Check sheet for the modelled part. Datum: model origin and axes. Units: mm. A direction names the side the tool comes from. Coordinates: 2 decimals unless noted, no trailing zeros. Loops run counter-clockwise (first coordinate to the right, second up) from the corner with the lowest first, then second, coordinate; pieces in that order, holes last. Notation, with made-up numbers: M 20,-20.75 L 28,-20.75 A22 cw 28,-9.75 Z; hole C 64,70 d10. An arc over 180 degrees is marked long. Use CSV: the item, a comma, the result in double quotes. Start each with the question number.
(1) Set-up check for faces 1 (the flat face through (8, 0, 0)), 2 (the flat face through (0, 3.1, -1.1)): record each of +Z, -Z, +X, -X, +Y, -Y from which the full face is reachable in a straight line by a thin tool's end or side.
(2) Section check A-A on z = 0. Record the cut outline in (x, y).
(3) Scan lines: line 1 (X direction, y = 3, z = -1.5); line 2 (Z direction, x = 3.5, y = 0); line 3 (X direction, y = -3.25, z = 3). Record each from-to range of solid material in increasing order.
(4) Draft check along Y on faces 3 (the flat face through (0, 0, 0)), 4 (the cylindrical face through (-0.33, 3.32, -3.04)), 5 (the flat face through (-1, -1, 1)). Enter one of: pulls with the +Y half, pulls with the -Y half, needs draft (parallel to the pull), parting line crosses it, or undercut.
(5) Go/stop test with flat-tipped pins: pin 1 Ø5 at (x, y) = (5.5, 0) entering from +Z; pin 2 Ø1.5 at (x, y) = (6.5, -3) entering from +Z; pin 3 Ø2 at (x, z) = (6, 3) entering from +Y. Record where each tip stops, or that it passes through.
(6) Section check C-C on x = 7.75. Record the cut outline in (y, z).
(7) Section check B-B on y = 0. Record the cut outline in (x, z) (3 decimals).
from build123d import *

# Parameters (mm, degrees)
CUT_EXTRUDE1_DEPTH = 1
FILLET1_R          = 0.6


with BuildPart() as part:
    # Sketch1 → Revolve1 (revolve)
    with BuildSketch(Plane.XY, mode=Mode.PRIVATE) as revolve1_sk:
        Polygon((0, 2.5), (8, 2.5), (8, 0), (-1, 0), (-1, 3.922649731), (-0.666666667, 4.5), (0, 4.5), align=None)
    revolve(revolve1_sk.sketch.rotate(Axis((-1, 0, 0), (1, 0, 0)), 180), axis=Axis((-1, 0, 0), (1, 0, 0)))

    # Sketch2 → Cut-Extrude1 (cut)
    with BuildSketch(Plane(origin=(-1, 0, 0), x_dir=(0, 0, -1), z_dir=(1, 0, 0))):
        with BuildLine():
            ThreePointArc((0.268841336, 1.198258139), (0, 1.4), (-0.268841336, 1.198258139))
            ThreePointArc((-0.268841336, 1.198258139), (-0.5125, 0.887676039), (-0.903301321, 0.831952496))
            ThreePointArc((-0.903301321, 0.831952496), (-1.212435565, 0.7), (-1.172142656, 0.366305643))
            ThreePointArc((-1.172142656, 0.366305643), (-1.025, 0), (-1.172142656, -0.366305643))
            ThreePointArc((-1.172142656, -0.366305643), (-1.212435565, -0.7), (-0.903301321, -0.831952496))
            ThreePointArc((-0.903301321, -0.831952496), (-0.5125, -0.887676039), (-0.268841336, -1.198258139))
            ThreePointArc((-0.268841336, -1.198258139), (0, -1.4), (0.268841336, -1.198258139))
            ThreePointArc((0.268841336, -1.198258139), (0.5125, -0.887676039), (0.903301321, -0.831952496))
            ThreePointArc((0.903301321, -0.831952496), (1.212435565, -0.7), (1.172142656, -0.366305643))
            ThreePointArc((1.172142656, -0.366305643), (1.025, 0), (1.172142656, 0.366305643))
            ThreePointArc((1.172142656, 0.366305643), (1.212435565, 0.7), (0.903301321, 0.831952496))
            ThreePointArc((0.903301321, 0.831952496), (0.5125, 0.887676039), (0.268841336, 1.198258139))
        make_face()
    extrude(amount=CUT_EXTRUDE1_DEPTH, mode=Mode.SUBTRACT)

    # Fillet1
    fillet1_edges = [part.edges().sort_by_distance(p)[0] for p in [
        (0, 2.5, 0),
    ]]
    fillet(fillet1_edges, radius=FILLET1_R)


solid = part.part
Outcome:
1,face 1,"+Z, -Z, +X, +Y, -Y"
1,face 2,"+X"
2,outline,"M -1,-3.92 L -0.67,-4.5 L 0,-4.5 L 0,-3.1 A0.6 cw 0.6,-2.5 L 8,-2.5 L 8,2.5 L 0.6,2.5 A0.6 cw 0,3.1 L 0,4.5 L -0.67,4.5 L -1,3.92 L -1,1.4 L 0,1.4 L 0,-1.4 L -1,-1.4 Z"
3,line 1,"x = -1 to 0"
3,line 2,"z = -2.5 to 2.5"
3,line 3,"x = -0.71 to 0"
4,face 3,"undercut"
4,face 4,"parting line crosses it"
4,face 5,"needs draft"
5,pin 1,"stops at z = 2.5"
5,pin 2,"stops at z = 1.09"
5,pin 3,"stops at y = 1.5"
6,outline,"C 0,0 d5"
7,outline,"M -1,-3.923 L -0.667,-4.5 L 0,-4.5 L 0,-3.1 A0.6 cw 0.6,-2.5 L 8,-2.5 L 8,2.5 L 0.6,2.5 A0.6 cw 0,3.1 L 0,4.5 L -0.667,4.5 L -1,3.923 L -1,1.025 L 0,1.025 L 0,-1.025 L -1,-1.025 Z"
